from build123d import *

# Parameters (mm, degrees)
FLANGE_BASE1_DEPTH    = 15
ESBO_O3_R             = 2
CORTE_EXTRUS_O2_DEPTH = 10


# Sheet-metal steps are written as plain solids
with BuildPart() as part:
    # Esboço1 → Flange-base1 (new body)
    with BuildSketch(Plane.XY):
        with BuildLine():
            Line((-19.5, 0), (-9, 0))
            ThreePointArc((-9, 0), (-7.939339828, 0.439339828), (-7.5, 1.5))
            Line((-7.5, 1.5), (-7.5, 17.5))
            ThreePointArc((-7.5, 17.5), (-7.353553391, 17.853553391), (-7, 18))
            Line((-7, 18), (7, 18))
            ThreePointArc((7, 18), (7.353553391, 17.853553391), (7.5, 17.5))
            Line((7.5, 17.5), (7.5, 1.5))
            ThreePointArc((7.5, 1.5), (7.939339828, 0.439339828), (9, 0))
            Line((9, 0), (19.5, 0))
            Line((19.5, 0), (19.5, 1))
            Line((19.5, 1), (9, 1))
            ThreePointArc((9, 1), (8.646446609, 1.146446609), (8.5, 1.5))
            Line((8.5, 1.5), (8.5, 17.5))
            ThreePointArc((8.5, 17.5), (8.060660172, 18.560660172), (7, 19))
            Line((7, 19), (-7, 19))
            ThreePointArc((-7, 19), (-8.060660172, 18.560660172), (-8.5, 17.5))
            Line((-8.5, 17.5), (-8.5, 1.5))
            ThreePointArc((-8.5, 1.5), (-8.646446609, 1.146446609), (-9, 1))
            Line((-9, 1), (-19.5, 1))
            Line((-19.5, 1), (-19.5, 0))
        make_face()
    extrude(amount=FLANGE_BASE1_DEPTH)

    # Esboço3 → Corte-extrusão2 (cut)
    with BuildSketch(Plane(origin=(0, 1, 0), x_dir=(1, 0, 0), z_dir=(0, 1, 0))):
        with Locations(Location((-14.25, -7.5, 0), (0, 0, 270))):
            Circle(ESBO_O3_R)
        with Locations(Location((14.25, -7.5, 0), (0, 0, 270))):
            Circle(ESBO_O3_R)
    extrude(amount=-CORTE_EXTRUS_O2_DEPTH, mode=Mode.SUBTRACT)


solid = part.part
Design review of the part built by this model. Coordinates are the model's own, in mm. A direction names the side the tool comes from. Coordinates: 2 decimals unless noted, no trailing zeros. Loops run counter-clockwise (first coordinate to the right, second up) from the corner with the lowest first, then second, coordinate; pieces in that order, holes last. Notation, with made-up numbers: (3.5, -8.5) -> (32.5, -8.5) arc R19 ccw to (32.5, 15.5) -> close; hole circle Ø11 at (-16, -4). An arc over 180 degrees is marked (long way). Use a Markdown table: item, result. Add a question column.
Item 1: Wall thickness on L1, parallel to X at y = 0.75, z = 7.5; L2, parallel to X at y = 16.5, z = 13.25; L3, parallel to X at y = 0.4, z = 7.5: over which ranges is each line inside the solid? List them lowest first. Write a range as from..to.
Item 2: We need section B-B, the plane y = 10. Write out the cut boundary in (x, z), and give its area (3 significant figures).
Item 3: We need section C-C, the plane z = 7.5. Write out the cut boundary in (x, y).
Item 4: Clearance check with flat-ended pins moving along their axes: P1, Ø5, axis at x = -13.5, z = 10, coming from the +Y side; P2, Ø7.5, axis at y = 6, z = 11, coming from the -X side; P3, Ø1.5, axis at y = 2.5, z = 12.5, coming from the +X side; P4, Ø2, axis at x = 2, y = 16.5, coming from the +Z side. State where each tip first meets the part, or that it passes through.
Item 5: The part is to be moulded in two halves that separate along Z. For faces 4 (the cylindrical face through (16.233, 0.507, 7.24)), 5 (the flat face through (-0.1, 18.7, 0)), 6 (the flat face through (-15.5, 0, 5.7)), say which applies: +Z half, -Z half, draft (parallel to the pull), parting line (faces both ways), or undercut.
Item 6: We need section A-A, the plane x = -14.25. Write out the cut boundary in (y, z), and give its area (3 significant figures).
Item 7: Machinability: for faces 1 (the flat face through (0, 18, 7)), 2 (the flat face through (-8.5, 10, 7)), 3 (the flat face through (15.5, 1, 5.7)), which of the approach directions +Z, -Z, +X, -X, +Y, -Y give a long, thin tool a straight path to every point of the face, cutting with its end or side? Answer none if there is none.
Item 8: We need section D-D, the plane z = 12.25. Write out the cut boundary in (x, y).
Numbers:
| question | item | result |
|---|---|---|
| 1 | L1 | x = -19.5..-16.25, -12.25..-7.7, 7.7..12.25, 16.25..19.5 |
| 1 | L2 | x = -8.5..-7.5, 7.5..8.5 |
| 1 | L3 | x = -19.5..-16.25, -12.25..-7.98, 7.98..12.25, 16.25..19.5 |
| 2 | outline | (-8.5, 0) -> (-7.5, 0) -> (-7.5, 15) -> (-8.5, 15) -> close; (7.5, 0) -> (8.5, 0) -> (8.5, 15) -> (7.5, 15) -> close |
| 2 | area | 30.0 mm^2 |
| 3 | outline | (-19.5, 0) -> (-16.25, 0) -> (-16.25, 1) -> (-19.5, 1) -> close; (-12.25, 0) -> (-9, 0) arc R1.5 ccw to (-7.5, 1.5) -> (-7.5, 17.5) arc R0.5 cw to (-7, 18) -> (7, 18) arc R0.5 cw to (7.5, 17.5) -> (7.5, 1.5) arc R1.5 ccw to (9, 0) -> (12.25, 0) -> (12.25, 1) -> (9, 1) arc R0.5 cw to (8.5, 1.5) -> (8.5, 17.5) arc R1.5 ccw to (7, 19) -> (-7, 19) arc R1.5 ccw to (-8.5, 17.5) -> (-8.5, 1.5) arc R0.5 cw to (-9, 1) -> (-12.25, 1) -> close; (16.25, 0) -> (19.5, 0) -> (19.5, 1) -> (16.25, 1) -> close |
| 4 | P1 | stops at y = 1 |
| 4 | P2 | stops at x = -8.5 |
| 4 | P3 | stops at x = 8.5 |
| 4 | P4 | passes through |
| 5 | face 4 | undercut |
| 5 | face 5 | -Z half |
| 5 | face 6 | draft |
| 6 | outline | (0, 0) -> (1, 0) -> (1, 5.5) -> (0, 5.5) -> close; (0, 9.5) -> (1, 9.5) -> (1, 15) -> (0, 15) -> close |
| 6 | area | 11.0 mm^2 |
| 7 | face 1 | +Z, -Z, -Y |
| 7 | face 2 | +Z, -Z, -X, +Y |
| 7 | face 3 | +Z, -Z, +X, +Y |
| 8 | outline | (-19.5, 0) -> (-9, 0) arc R1.5 ccw to (-7.5, 1.5) -> (-7.5, 17.5) arc R0.5 cw to (-7, 18) -> (7, 18) arc R0.5 cw to (7.5, 17.5) -> (7.5, 1.5) arc R1.5 ccw to (9, 0) -> (19.5, 0) -> (19.5, 1) -> (9, 1) arc R0.5 cw to (8.5, 1.5) -> (8.5, 17.5) arc R1.5 ccw to (7, 19) -> (-7, 19) arc R1.5 ccw to (-8.5, 17.5) -> (-8.5, 1.5) arc R0.5 cw to (-9, 1) -> (-19.5, 1) -> close |
